For this review, take the finished solid that the model builds, in its own axes (mm). Face numbers are marked on the shaded views. A direction names the side the tool comes from. Round coordinates to 2 decimals unless told otherwise and drop trailing zeros. Write each loop counter-clockwise with the first axis right and the second up, starting at its lowest first coordinate (ties: lowest second). Pieces come first, ordered by that corner, then holes. Notation, with made-up numbers: (51, 89) - (76, 89) arc R13 ccw to (76, 110) - close; hole circle Ø3 at (-14.5, 0). An arc over 180 degrees is marked (long way). One line per item, written item: value. Start each with the question number.
Q1. Add section A-A on y = 6.35. Write out the cut boundary in (x, z).
Q2. Add section B-B on x = 38.1. Write out the cut boundary in (y, z).
Q3. Add section D-D on x = -10.5. Write out the cut boundary in (y, z), and give its area (3 significant figures).
Q4. Add section C-C on z = -4. Write out the cut boundary in (x, y).
Q5. Tool access review of the marked faces 1 and 2: name each direction out of +Z, -Z, +X, -X, +Y, -Y from which nothing blocks a thin tool from reaching the whole face with its end or side.
Q6. Clearance check with flat-ended pins moving along their axes: pin 1 Ø4 at (x, z) = (-20.5, 9) entering from +Y; pin 2 Ø1 at (x, z) = (-0.5, -4.5) entering from -Y; pin 3 Ø3 at (x, y) = (-6, 7) entering from -Z; pin 4 Ø5 at (y, z) = (6.5, 0) entering from -X. State where each tip first meets the part, or that it passes through.
Q7. For probe 1 along Y at (x, z) = (38.1, 11.8); probe 2 along Y at (x, z) = (10.5, 2); probe 3 along Z at (x, y) = (-9, 7), list the stretches that pass through material, from the lowest coordinate up.
Autodesk Inventor part; units mm, degrees
ref_plane "YZ Plane" through (0, 0, 0) normal (1, 0, 0) x (0, 1, 0)
ref_plane "XZ Plane" through (0, 0, 0) normal (0, 1, 0) x (-1, 0, 0)
ref_plane "XY Plane" through (0, 0, 0) normal (0, 0, 1) x (1, 0, 0)
sketch "Sketch1" plane through (0, 0, 0) normal (0, 1, 0) x (-1, 0, 0)
  line L0 (-44.45, 12.7) -> (44.45, 12.7)
  line L1 (44.45, 12.7) -> (44.45, -12.7)
  line L2 (44.45, -12.7) -> (-44.45, -12.7)
  line L3 (-44.45, -12.7) -> (-44.45, 12.7)
  line L4 (-44.45, 12.7) -> (44.45, -12.7) construction
  line L5 (44.45, 12.7) -> (-44.45, -12.7) construction
  point P0 (0, 0)
  dimension "d0" = 88.9
  dimension "d1" = 25.4
extrude "Extrusion1" add sketch "Sketch1" along normal blind 1.5875
sketch "Sketch2" plane through (0, 1.5875, 0) normal (0, 1, 0) x (1, 0, 0)
  line L0 (-44.45, -12.7) -> (44.45, -12.7)
  line L1 (-44.45, -12.7) -> (-44.45, -11.1125)
  line L2 (-44.45, 12.7) -> (-44.45, -12.7)
  line L3 (-44.45, -11.1125) -> (44.45, -11.1125)
  line L4 (44.45, -11.1125) -> (44.45, -12.7)
  line L5 (44.45, -12.7) -> (-44.45, -12.7)
  line L6 (-44.45, -12.7) -> (-44.45, -11.1125)
  point P0 (0, 0)
  dimension "d4" = 1.5875
extrude "Extrusion2" add sketch "Sketch2" along normal blind 9.525
sketch "Sketch3" plane through (44.45, 1.5875, 11.1125) normal (0, 0, -1) x (-1, 0, 0)
  line L0 (0, -1.5875) -> (0, 9.525)
  line L1 (0, 9.525) -> (6.35, 9.525)
  line L2 (88.9, 9.525) -> (0, 9.525)
  line L3 (88.9, 0) -> (0, 0)
  line L4 (88.9, 0) -> (88.9, 9.525)
  line L5 (0, 9.525) -> (88.9, 9.525)
  line L6 (0, 0) -> (0, 9.525)
  line L7 (0, 0) -> (88.9, 0)
  line L8 (6.35, 9.525) -> (6.35, 4.7625)
  circle A0 centre (6.35, 4.7625) radius 1.4351
  point P0 (44.45, -1.5875)
  dimension "d7" = 6.35
  dimension "d8" = 2.8702
extrude "Extrusion3" cut sketch "Sketch3" against normal through all contours A0
properties part number "Switch-Panel-Divider"
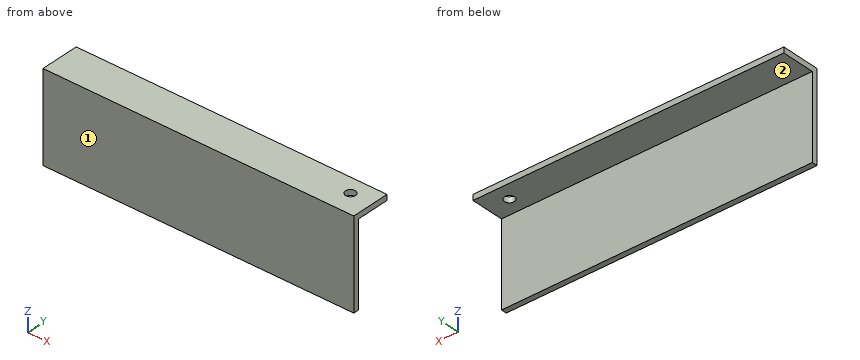
Result set:
1. outline: (-44.45, 11.11) - (36.66, 11.11) - (36.66, 12.7) - (-44.45, 12.7) - close; (39.54, 11.11) - (44.45, 11.11) - (44.45, 12.7) - (39.54, 12.7) - close
2. outline: (0, -12.7) - (1.59, -12.7) - (1.59, 11.11) - (4.91, 11.11) - (4.91, 12.7) - (0, 12.7) - close; (7.79, 11.11) - (11.11, 11.11) - (11.11, 12.7) - (7.79, 12.7) - close
3. outline: (0, -12.7) - (1.59, -12.7) - (1.59, 11.11) - (11.11, 11.11) - (11.11, 12.7) - (0, 12.7) - close
3. area: 55.4 mm^2
4. outline: (-44.45, 0) - (44.45, 0) - (44.45, 1.59) - (-44.45, 1.59) - close
5. face 1: +Z, -Z, +X, -X, -Y
5. face 2: -Z, +X, -X, +Y
6. pin 1: stops at y = 1.59
6. pin 2: stops at y = 0
6. pin 3: stops at z = 11.11
6. pin 4: passes through
7. probe 1: y = 0 to 4.91, 7.79 to 11.11
7. probe 2: y = 0 to 1.59
7. probe 3: z = 11.11 to 12.7
